Input: part model. Units: mm. Frame: model coordinates. A direction names the side the tool comes from. Round coordinates to 2 decimals unless told otherwise and drop trailing zeros. Write each loop counter-clockwise with the first axis right and the second up, starting at its lowest first coordinate (ties: lowest second). Pieces come first, ordered by that corner, then holes. Notation, with made-up numbers: (5, -40) - (29, -40) arc R21 cw to (29, -32) - close; hole circle Ø8 at (83, 66). An arc over 180 degrees is marked (long way). Use one line per item in the form item = value.
```python
from build123d import *

# Parameters (mm, degrees)
CYLINDER_R     = 18.5
CYLINDER_DEPTH = 10
BOX001_W       = 10
BOX001_H       = 10
BOX001_DEPTH   = 10
BOX_W          = 57
BOX_H          = 47
BOX_DEPTH      = 10


with BuildPart() as cylinder:
    # Cylinder → Cylinder (new body)
    with BuildSketch(Plane(origin=(18.5, 0, -5), x_dir=(1, 0, 0), z_dir=(0, 0, 1))):
        Circle(CYLINDER_R)
    extrude(amount=CYLINDER_DEPTH)


with BuildPart() as fusion:
    # Box001 → Box001 (new body)
    with BuildSketch(Plane(origin=(-5, -5, -5), x_dir=(1, 0, 0), z_dir=(0, 0, 1))):
        with Locations((5, 5)):
            Rectangle(BOX001_W, BOX001_H)
    extrude(amount=BOX001_DEPTH)

    # Fusion: union Cylinder
    add(cylinder.part)


with BuildPart() as cut:
    # Box → Box (new body)
    with BuildSketch(Plane(origin=(-10, -23.5, -5), x_dir=(1, 0, 0), z_dir=(0, 0, 1))):
        with Locations((28.5, 23.5)):
            Rectangle(BOX_W, BOX_H)
    extrude(amount=BOX_DEPTH)

    # Cut: cut Fusion
    add(fusion.part, mode=Mode.SUBTRACT)


solid = cut.part
```
(1) Cut plane C-C on y = 0. Output: boundary loops of the cut face in (x, z), then the cut area to 3 significant figures.
Derived:
outline = (-10, -5) - (-5, -5) - (-5, 5) - (-10, 5) - close; (37, -5) - (47, -5) - (47, 5) - (37, 5) - close
area = 150 mm^2
(2) Cut plane B-B on z = 0. Output: boundary loops of the cut face in (x, y).
Derived:
outline = (-10, -23.5) - (47, -23.5) - (47, 23.5) - (-10, 23.5) - close; hole (-5, -5) - (0.69, -5) arc R18.5 ccw (long way) to (0.69, 5) - (-5, 5) - close
(3) Access query for faces 1 (the face through (-5, 0, 0)), 2 (the face through (37, 6, -5)). Directions: +Z, -Z, +X, -X, +Y, -Y. A direction counts if a zero-diameter tool reaches every point of the face in a straight line with its end or side. Return the directions, or none.
Derived:
face_1 = +Z, -Z
face_2 = -Z, +X, -X, +Y, -Y
(4) Material intervals for L1, parallel to Y at x = 18.5, z = -2.75; L2, parallel to X at y = 0, z = -2.5; L3, parallel to Y at x = -0.5, z = -0.25, sorted ascending.
Derived:
L1 = -23.5 to -18.5, 18.5 to 23.5
L2 = -10 to -5, 37 to 47
L3 = -23.5 to -5, 5 to 23.5
(5) Draft query along X for faces 3 (the face through (-2, 5, 0)), 4 (the face through (-10, 0, 0)), 5 (the face through (18, -23.5, 0)). Return one class per face: released by +X, released by -X, zero draft, split by the parting line, or undercut.
Derived:
face_3 = undercut
face_4 = released by -X
face_5 = zero draft
(6) Cut plane A-A on x = 18.5. Output: boundary loops of the cut face in (y, z).
Derived:
outline = (-23.5, -5) - (-18.5, -5) - (-18.5, 5) - (-23.5, 5) - close; (18.5, -5) - (23.5, -5) - (23.5, 5) - (18.5, 5) - close
